CAD build for the part. Positions are in the model's coordinates, mm. Face numbers are marked on the shaded views. A direction names the side the tool comes from. Round coordinates to 2 decimals unless told otherwise and drop trailing zeros. Write each loop counter-clockwise with the first axis right and the second up, starting at its lowest first coordinate (ties: lowest second). Pieces come first, ordered by that corner, then holes. Notation, with made-up numbers: (-15.5, 64) - (31.5, 64) arc R25 ccw to (31.5, 87) - close; hole circle Ø1 at (-39.75, 75). An arc over 180 degrees is marked (long way). Use one line per item in the form item = value. Start each with the question number.
Item 1: Band-saw the part on D-D, the plane z = 31.5. List the corners of the cut face in (x, y).
Item 2: Band-saw the part on B-B, the plane y = 1.5. Give the number of separate pieces and of enclosed holes in the cut face, and give its area (3 significant figures).
Item 3: Pin check, flat tips, straight feed: pin 1 (5 mm diameter, centred on x = -53.5, z = -9, fed in from -Y); pin 2 (3.5 mm diameter, centred on x = -79, z = 17.5, fed in from +Y); pin 3 (3 mm diameter, centred on y = -38.5, z = 19.5, fed in from -X). Stop position of each tip, or through.
Item 4: Drill centre lines: L1, parallel to X at y = 6.75, z = -19; L2, parallel to Z at x = -81.25, y = 13.25; L3, parallel to X at y = -29, z = 19. Where is each one in solid material? Low to high.
Item 5: Band-saw the part on C-C, the plane x = 27.75. List the corners of the cut face in (y, z) (3 decimals).
Item 6: Tool access for the marked faces 1 and 2: list every direction of +Z, -Z, +X, -X, +Y, -Y with a clear straight run to the whole face (end or side of a thin tool).
Item 7: Band-saw the part on A-A, the plane x = -40.25. List the corners of the cut face in (y, z).
from build123d import *

# Parameters (mm, degrees)
BOSS_EXTRUDE1_DEPTH  = 43
M6_CLEARANCE_HOLE1_D = 7
SKETCH4_R            = 5.5
CUT_EXTRUDE1_DEPTH   = 7
SKETCH5_W            = 10.25
SKETCH5_H            = 5.25
CUT_EXTRUDE2_DEPTH   = 22
SKETCH6_W            = 10.5
SKETCH6_H            = 5.25
CUT_EXTRUDE3_DEPTH   = 32
FILLET1_R            = 2.5


with BuildPart() as part:
    # Sketch1 → Boss-Extrude1 (new, symmetric)
    with BuildSketch(Plane.XY):
        Polygon((0, 0), (0, -44.7), (41, -44.7), (41, 15.25), (-94.5, 15.25), (-94.5, 0), align=None)
    extrude(amount=BOSS_EXTRUDE1_DEPTH, both=True)

    # M6 Clearance Hole1 (through all)
    with Locations(Plane(origin=(0, 15.25, 0), x_dir=(1, 0, 0), z_dir=(0, 1, 0))):
        with Locations((-81.25, 19), (-81.25, -19), (-13.25, -19), (-13.25, 19), (27.75, 19), (27.75, -19), (-40.25, 19), (-40.25, -19)):
            Hole(M6_CLEARANCE_HOLE1_D / 2)

    # Sketch4 → Cut-Extrude1 (cut)
    with BuildSketch(Plane(origin=(0, 15.25, 0), x_dir=(1, 0, 0), z_dir=(0, 1, 0))):
        with Locations(Location((-81.25, 19, 0), (0, 0, 180))):
            Circle(SKETCH4_R)
        with Locations(Location((-81.25, -19, 0), (0, 0, 180))):
            Circle(SKETCH4_R)
        with Locations(Location((-13.25, 19, 0), (0, 0, 180))):
            Circle(SKETCH4_R)
        with Locations(Location((-13.25, -19, 0), (0, 0, 180))):
            Circle(SKETCH4_R)
    extrude(amount=-CUT_EXTRUDE1_DEPTH, mode=Mode.SUBTRACT)

    # Sketch5 → Cut-Extrude2 (cut)
    with BuildSketch(Plane(origin=(41, 0, 0), x_dir=(0, 0, -1), z_dir=(1, 0, 0))):
        with Locations((-19, -7.625)):
            Rectangle(SKETCH5_W, SKETCH5_H)
        with Locations((19, -7.625)):
            Rectangle(SKETCH5_W, SKETCH5_H)
    extrude(amount=-CUT_EXTRUDE2_DEPTH, mode=Mode.SUBTRACT)

    # Sketch6 → Cut-Extrude3 (cut)
    with BuildSketch(Plane.XY.offset(43)):
        with Locations((-40.25, 9.625)):
            Rectangle(SKETCH6_W, SKETCH6_H)
    cut_extrude3 = extrude(amount=-CUT_EXTRUDE3_DEPTH, mode=Mode.SUBTRACT)

    # Mirror1: Cut-Extrude3 across plane
    add(cut_extrude3.mirror(Plane.XY), mode=Mode.SUBTRACT)

    # Fillet1
    fillet1_edges = [part.edges().sort_by_distance(p)[0] for p in [
        (41, -14.725, 43),
        (-94.5, 7.625, 43),
        (-94.5, 7.625, -43),
        (41, -14.725, -43),
        (0, -22.35, -43),
        (0, -22.35, 43),
    ]]
    fillet(fillet1_edges, radius=FILLET1_R)


solid = part.part
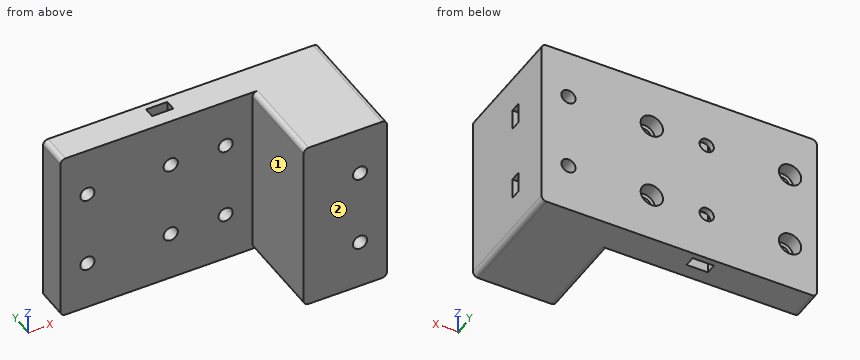
Determined:
q1.outline = (-94.5, 0) - (0, 0) - (0, -44.7) - (41, -44.7) - (41, 15.25) - (-94.5, 15.25) - close; hole (-45.5, 7) - (-35, 7) - (-35, 12.25) - (-45.5, 12.25) - close
q2.separate_pieces = 1
q2.enclosed_holes = 8
q2.area = 11,300 mm²
q3.pin_1 = 0
q3.pin_2 = 8.25
q3.pin_3 = 0
q4.L1 = -94.5 to -84.75, -77.75 to -43.75, -36.75 to -16.75, -9.75 to 24.25, 31.25 to 41
q4.L2 = -43 to -24.5, -13.5 to 13.5, 24.5 to 43
q4.L3 = 0 to 24.25, 31.25 to 41
q5.outline = (-44.7, -43) - (15.25, -43) - (15.25, -22.5) - (-5, -22.5) - (-5, -24.125) - (-10.25, -24.125) - (-10.25, -22.5) - (-44.7, -22.5) - close; (-44.7, -15.5) - (-10.25, -15.5) - (-10.25, -13.875) - (-5, -13.875) - (-5, -15.5) - (15.25, -15.5) - (15.25, 15.5) - (-5, 15.5) - (-5, 13.875) - (-10.25, 13.875) - (-10.25, 15.5) - (-44.7, 15.5) - close; (-44.7, 22.5) - (-10.25, 22.5) - (-10.25, 24.125) - (-5, 24.125) - (-5, 22.5) - (15.25, 22.5) - (15.25, 43) - (-44.7, 43) - close
q6.face_1 = +Z, -Z, -X, -Y
q6.face_2 = +Z, -Z, +X, -X, -Y
q7.outline = (0, -43) - (7, -43) - (7, -22.5) - (0, -22.5) - close; (0, -15.5) - (7, -15.5) - (7, -11) - (12.25, -11) - (12.25, -15.5) - (15.25, -15.5) - (15.25, 15.5) - (12.25, 15.5) - (12.25, 11) - (7, 11) - (7, 15.5) - (0, 15.5) - close; (0, 22.5) - (7, 22.5) - (7, 43) - (0, 43) - close; (12.25, -43) - (15.25, -43) - (15.25, -22.5) - (12.25, -22.5) - close; (12.25, 22.5) - (15.25, 22.5) - (15.25, 43) - (12.25, 43) - close
